Autodesk Fusion 360 part; units mm, degrees
sketch "Sorted Smarties Top" plane through (0, 0, 0) normal (0, 0, 1) x (1, 0, 0)
  line L0 (0, 0) -> (-270, 0)
  line L1 (-270, 0) -> (-270, 94)
  line L2 (-270, 94) -> (0, 94)
  line L3 (0, 94) -> (0, 0)
  dimension "d2" = 270
  dimension "d3" = 94
extrude "Extrude1" add sketch "Sorted Smarties Top" along normal blind 6
sketch "Sketch2" plane through (0, 0, 0) normal (0, 0, -1) x (1, 0, 0)
  line L0 (-270, -94) -> (0, -94)
  line L1 (0, -94) -> (0, 0)
  line L2 (0, 0) -> (-270, 0)
  line L3 (-270, 0) -> (-270, -94)
  line L4 (-5, -10) -> (-265, -10)
  line L5 (-265, -10) -> (-265, -20)
  line L6 (-265, -20) -> (-5, -20)
  line L7 (-5, -20) -> (-5, -10)
  line L8 (-5, -45) -> (-265, -45)
  line L9 (-265, -45) -> (-265, -55)
  line L10 (-265, -55) -> (-5, -55)
  line L11 (-5, -55) -> (-5, -45)
  dimension "d6" = 10
  dimension "d7" = 10
  dimension "d8" = 10
  dimension "d9" = 25
  dimension "d10" = 5
  dimension "d11" = 5
  dimension "d12" = 5
  dimension "d13" = 5
extrude "Extrude2" cut sketch "Sketch2" against normal blind 4 contours L4 L5 L6 L7 | L8 L9 L10 L11
sketch "Sketch3" plane through (0, 0, 4) normal (0, 0, -1) x (1, 0, 0)
  line L0 (-5, -20) -> (-5, -10)
  line L1 (-5, -10) -> (-265, -10)
  line L2 (-265, -10) -> (-265, -20)
  line L3 (-265, -20) -> (-5, -20)
  line L4 (-5, -10) -> (-15, -10)
  line L5 (-15, -10) -> (-15, -20)
  line L6 (-15, -20) -> (-5, -20)
  line L7 (-5, -20) -> (-5, -10)
  line L8 (-5, -45) -> (-15, -45)
  line L9 (-15, -45) -> (-15, -55)
  line L10 (-15, -55) -> (-5, -55)
  line L11 (-5, -55) -> (-5, -45)
extrude "Extrude3" cut sketch "Sketch3" against normal blind 2 contours L0 L1 L3 L4 L5 L6 L7 | L8 L9 L10 L11
equation "MDFThickness = 6 mm"
equation "d3 = 100 mm - MDFThickness"
equation "d4 = MDFThickness"
Source: CAD feature listing. Evaluate the final solid. Frame: model axes, mm. A direction names the side the tool comes from. Coordinates: 2 decimals unless noted, no trailing zeros. Write each loop counter-clockwise with the first axis right and the second up, starting at its lowest first coordinate (ties: lowest second). Pieces come first, ordered by that corner, then holes. Notation, with made-up numbers: M 75.5,72 L 105.5,72 A18 ccw 105.5,98 Z; hole C -18.75,8.5 d4. An arc over 180 degrees is marked long. Answer as a JSON object with one key per item and string values.
1. Ray query, L1, parallel to Y at x = -74, z = 2.9; L2, parallel to X at y = 54, z = 5.8; L3, parallel to X at y = 13, z = 3.5. Return the intervals inside material, ascending.
Evaluation:
{"L1": "0 to 10, 20 to 45, 55 to 94", "L2": "-270 to -15, -5 to 0", "L3": "-270 to -265, -5 to 0"}
2. Cut plane A-A on y = 16. Output: boundary loops of the cut face in (x, z), plus the area to 3 significant figures.
Evaluation:
{"outline": "M -270,0 L -265,0 L -265,4 L -15,4 L -15,6 L -270,6 Z; M -5,0 L 0,0 L 0,6 L -5,6 Z", "area": "560 mm^2"}
3. Cut plane B-B on z = 3.05. Output: boundary loops of the cut face in (x, y).
Evaluation:
{"outline": "M -270,0 L 0,0 L 0,94 L -270,94 Z; hole M -265,10 L -5,10 L -5,20 L -265,20 Z; hole M -265,45 L -5,45 L -5,55 L -265,55 Z"}
4. Contact query for a flat-ended pin moving along its axis: P1, Ø5, axis at x = -140.5, y = 14, coming from the -Z side. Output: stop coordinate, or through.
Evaluation:
{"P1": "z = 4"}
5. Cut plane C-C on x = -27. Output: boundary loops of the cut face in (y, z).
Evaluation:
{"outline": "M 0,0 L 10,0 L 10,4 L 20,4 L 20,0 L 45,0 L 45,4 L 55,4 L 55,0 L 94,0 L 94,6 L 0,6 Z"}
6. Draft query along Y for faces 4 (the flat face through (-142, 15, 4)), 5 (the flat face through (-137, 94, 3)), 6 (the flat face through (-137, 58, 0)). Return one class per face: released by +Y, released by -Y, zero draft, split by the parting line, or undercut.
Evaluation:
{"face 4": "undercut", "face 5": "released by +Y", "face 6": "zero draft"}
7. Access query for faces 1 (the flat face through (-5, 50, 3)), 2 (the flat face through (-137, 55, 2)), 3 (the flat face through (-270, 46, 3)). Directions: +Z, -Z, +X, -X, +Y, -Y. A direction counts if a zero-diameter tool reaches every point of the face in a straight line with its end or side. Return the directions, or none.
Evaluation:
{"face 1": "+Z, -Z", "face 2": "-Z", "face 3": "+Z, -Z, -X, +Y, -Y"}
